```python
from build123d import *

# Parameters (mm, degrees)
F0_W           = 114.3
F0_H           = 41.275
F1_DEPTH       = 12.7
F3_D           = 5.1054
F3_CSINK_D     = 10.4394
F3_CSINK_ANGLE = 82
F5_D           = 4.0386
F5_DEPTH       = 19.05
F5_TIP         = 1.213317848
F6_W           = 98.425
F6_H           = 3.175
F7_DEPTH       = 3.175
F9_DEPTH       = 6.35


with BuildPart() as f1:
    # F0 (on Front) → F1 (new body)
    with BuildSketch(Plane.XZ):
        Rectangle(F0_W, F0_H)
    extrude(amount=F1_DEPTH)

    # F3 (through all)
    with Locations(Plane.XZ.offset(12.7)):
        with Locations((50.8, 11.1125), (50.8, -11.1125), (-23.2833333333, -14.2875), (10.5833333333, -14.2875)):
            CounterSinkHole(F3_D / 2, F3_CSINK_D / 2, counter_sink_angle=F3_CSINK_ANGLE)

    # F5
    with Locations(Plane(origin=(-57.15, 0, 0), x_dir=(0, -1, 0), z_dir=(-1, 0, 0))):
        with Locations((6.35, 11.1125), (6.35, -11.1125)):
            Hole(F5_D / 2, depth=F5_DEPTH)
            with Locations((0, 0, -(F5_DEPTH + F5_TIP / 2))):  # 118° drill point
                Cone(0, F5_D / 2, F5_TIP, mode=Mode.SUBTRACT)

    # F6 (on face) → F7 (join)
    with BuildSketch(Plane(origin=(0, 0, 0), x_dir=(-1, 0, 0), z_dir=(0, 1, 0))):
        with Locations((4.7625, 19.05)):
            Rectangle(F6_W, F6_H)
    extrude(amount=F7_DEPTH)

    # F8 (on face) → F9 (cut)
    with BuildSketch(Plane.XZ.offset(12.7)):
        with BuildLine():
            Line((39.6744738062, 14.2875), (-50.8, 14.2875))
            Line((-50.8, 14.2875), (-50.8, -14.2875))
            Line((-50.8, -14.2875), (-34.8530333333, -14.2875))
            ThreePointArc((-34.8530333333, -14.2875), (-23.2833333333, -2.7178), (-11.7136333333, -14.2875))
            Line((-11.7136333333, -14.2875), (-0.9863666667, -14.2875))
            ThreePointArc((-0.9863666667, -14.2875), (10.5833333333, -2.7178), (22.1530333333, -14.2875))
            Line((22.1530333333, -14.2875), (39.6744738062, -14.2875))
            ThreePointArc((39.6744738062, -14.2875), (40.6765711012, -5.5112371584), (47.5797046968, 0))
            ThreePointArc((47.5797046968, 0), (40.6765711012, 5.5112371584), (39.6744738062, 14.2875))
        make_face()
    extrude(amount=-F9_DEPTH, mode=Mode.SUBTRACT)


solid = f1.part
```
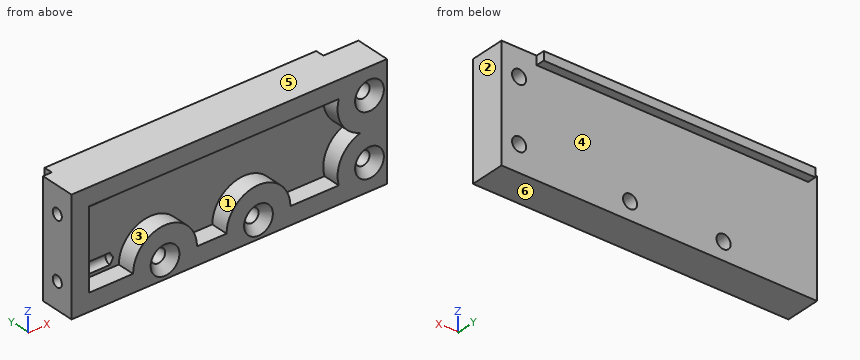
Verification items for the finished model (mm, model axes). Face numbers are marked on the shaded views. A direction names the side the tool comes from. Coordinates: 2 decimals unless noted, no trailing zeros. Loops run counter-clockwise (first coordinate to the right, second up) from the corner with the lowest first, then second, coordinate; pieces in that order, holes last. Notation, with made-up numbers: (79, -9) - (90, -9) arc R9 ccw to (90, -5) - close; hole circle Ø7 at (49, -5.5). An arc over 180 degrees is marked (long way). Put each result on its own line as item: value.
Item 1: Section check C-C (y = -1.75). Enter the section's corners in (x, z), then the cut area to 3 significant figures.
Conclusion:
outline: (-57.15, -20.64) - (57.15, -20.64) - (57.15, 20.64) - (-57.15, 20.64) - close; hole circle Ø5.11 at (-23.28, -14.29); hole circle Ø5.11 at (10.58, -14.29); hole circle Ø5.11 at (50.8, -11.11); hole circle Ø5.11 at (50.8, 11.11)
area: 4,640 mm2
Item 2: Section check A-A (x = 50.8). Enter the section's corners in (y, z).
Conclusion:
outline: (-12.7, -20.64) - (0, -20.64) - (0, -13.67) - (-9.63, -13.67) - (-12.7, -16.33) - close; (-12.7, -5.89) - (-9.63, -8.56) - (0, -8.56) - (0, 8.56) - (-9.63, 8.56) - (-12.7, 5.89) - close; (-12.7, 16.33) - (-9.63, 13.67) - (0, 13.67) - (0, 20.64) - (-12.7, 20.64) - close
Item 3: Gauge pin test, flat ends, axial feed: pin 1 Ø8.5 at (x, z) = (19.5, 1.5) entering from -Y; pin 2 Ø1.6 at (x, y) = (13, 1.5) entering from -Z; pin 3 Ø4.5 at (x, z) = (-23.28, -14.29) entering from -Y; pin 4 Ø2.5 at (y, z) = (2, 19) entering from +X. Record the tip position at first contact, or that the pin passes through.
Conclusion:
pin 1: stops at y = -6.35
pin 2: stops at z = 17.46
pin 3: passes through
pin 4: stops at x = 44.45
Item 4: Draft check along Z on the marked faces 3, 4, 5 and 6. Enter one of: pulls with the +Z half, pulls with the -Z half, needs draft (parallel to the pull), parting line crosses it, or undercut.
Conclusion:
face 3: undercut
face 4: needs draft
face 5: pulls with the +Z half
face 6: pulls with the -Z half
Item 5: Scan lines: line 1 along X through (y, z) = (-11.75, 10.5); line 2 along X through (y, z) = (-2, -16); line 3 along Y through (x, z) = (-24, 16). Record each from-to range of solid material in increasing order.
Conclusion:
line 1: x = -57.15 to -50.8, 39.25 to 46.45, 55.15 to 57.15
line 2: x = -57.15 to -25.18, -21.39 to 8.69, 12.48 to 57.15
line 3: y = -12.7 to 0
Item 6: Set-up check for the marked faces 1 and 2: record each of +Z, -Z, +X, -X, +Y, -Y from which the full face is reachable in a straight line by a thin tool's end or side.
Conclusion:
face 1: -Y
face 2: +Z, -Z, +X, +Y, -Y
